from build123d import *

# Parameters (mm, degrees)
SKETCH_1_W               = 20
SKETCH_1_H               = 24
EXTRUDE_1_DEPTH          = 24
CUT_EXTRUDE_1_DEPTH      = 24
SKETCH_3_W               = 10
SKETCH_3_H               = 5
CUT_EXTRUDE_2_DEPTH      = 20
EXTRUDE_2_DEPTH          = 10
SKETCH_5_W               = 10
SKETCH_5_H               = 16
EXTRUDE_3_DEPTH          = 6
FILLET_2_R               = 0.5
CHAMFER_3_SIZE           = 3
CHAMFER_4_SIZE           = 3
FILLET_3_R               = 1
CUT_EXTRUDE_3_REACH      = 24
CUT_EXTRUDE_3_END_RADIUS = 5
CUT_EXTRUDE_4_REACH      = 20
CUT_EXTRUDE_4_END_RADIUS = 5
FILLET_6_R               = 3
FILLET_7_R               = 3


with BuildPart() as part:
    # 草图1 → 拉伸1 (new body)
    with BuildSketch(Plane.XY):
        with Locations((10, 12)):
            Rectangle(SKETCH_1_W, SKETCH_1_H)
    extrude(amount=EXTRUDE_1_DEPTH)

    # 草图2 → 切除-拉伸1 (cut)
    with BuildSketch(Plane.XY.offset(24)):
        with BuildLine():
            Line((6.75, 15.75), (6.75, 8.25))
            ThreePointArc((6.75, 8.25), (10, 5), (13.25, 8.25))
            Line((13.25, 8.25), (13.25, 15.75))
            ThreePointArc((13.25, 15.75), (10, 19), (6.75, 15.75))
        make_face()
    extrude(amount=-CUT_EXTRUDE_1_DEPTH, mode=Mode.SUBTRACT)

    # 草图3 → 切除-拉伸2 (cut)
    with BuildSketch(Plane(origin=(0, 24, 0), x_dir=(1, 0, 0), z_dir=(0, 1, 0))):
        with Locations((10, -12.5)):
            Rectangle(SKETCH_3_W, SKETCH_3_H)
    extrude(amount=-CUT_EXTRUDE_2_DEPTH, mode=Mode.SUBTRACT)

    # 草图4 → 拉伸2 (add)
    with BuildSketch(Plane.XZ):
        with BuildLine():
            Line((15, 19), (10, 19))
            ThreePointArc((10, 19), (6.464466094, 17.535533906), (5, 14))
            Line((5, 14), (5, 9))
            Line((5, 9), (10, 9))
            ThreePointArc((10, 9), (13.535533906, 10.464466094), (15, 14))
            Line((15, 14), (15, 19))
        make_face()
    extrude(amount=EXTRUDE_2_DEPTH)

    # 草图5 → 拉伸3 (add)
    with BuildSketch(Plane.XZ.offset(10)):
        with Locations((10, 14)):
            Rectangle(SKETCH_5_W, SKETCH_5_H)
    extrude(amount=-EXTRUDE_3_DEPTH)

    # 圆角2
    fillet_2_edges = [part.edges().sort_by_distance(p)[0] for p in [
        (20, 12, 24),
        (0, 12, 24),
        (20, 12, 0),
        (0, 12, 0),
    ]]
    fillet(fillet_2_edges, radius=FILLET_2_R)

    # 倒角3
    chamfer_3_edges = [part.edges().sort_by_distance(p)[0] for p in [
        (10, -10, 22),
    ]]
    chamfer(chamfer_3_edges, length=CHAMFER_3_SIZE)

    # 倒角4
    chamfer_4_edges = [part.edges().sort_by_distance(p)[0] for p in [
        (10, -10, 6),
    ]]
    chamfer(chamfer_4_edges, length=CHAMFER_4_SIZE)

    # 圆角3
    fillet_3_edges = [part.edges().sort_by_distance(p)[0] for p in [
        (10, -10, 19),
        (10, -10, 9),
    ]]
    fillet(fillet_3_edges, radius=FILLET_3_R)

    # 切除-拉伸3: up to this cylinder (the profile starts outside it)
    cut_extrude_3_end = Plane(origin=(10, -4.087346, 14), z_dir=(0, 1, 0)) * Cylinder(CUT_EXTRUDE_3_END_RADIUS, 59, mode=Mode.PRIVATE)
    # 草图8 → 切除-拉伸3 (cut, up to the surface)
    with BuildSketch(Plane.XY.offset(22), mode=Mode.PRIVATE) as cut_extrude_3_sk1:
        Polygon((10, -4), (5, -4), (5, -4.262038896), align=None)
    cut_extrude_3_tool1 = extrude(cut_extrude_3_sk1.sketch, amount=-CUT_EXTRUDE_3_REACH, mode=Mode.PRIVATE) - cut_extrude_3_end
    add(cut_extrude_3_tool1.solids().sort_by_distance((6.666667, -4.087346, 22))[0], mode=Mode.SUBTRACT)

    # 切除-拉伸4: up to this cylinder (the profile starts outside it)
    cut_extrude_4_end = Plane(origin=(10, -4.087346, 14), z_dir=(0, 1, 0)) * Cylinder(CUT_EXTRUDE_4_END_RADIUS, 51, mode=Mode.PRIVATE)
    # 草图9 → 切除-拉伸4 (cut, up to the surface)
    with BuildSketch(Plane(origin=(0, 0, 6), x_dir=(-1, 0, 0), z_dir=(0, 0, -1)), mode=Mode.PRIVATE) as cut_extrude_4_sk1:
        Polygon((-10, -4), (-15, -4), (-15, -4.262038896), align=None)
    cut_extrude_4_tool1 = extrude(cut_extrude_4_sk1.sketch, amount=-CUT_EXTRUDE_4_REACH, mode=Mode.PRIVATE) - cut_extrude_4_end
    add(cut_extrude_4_tool1.solids().sort_by_distance((13.333333, -4.087346, 6))[0], mode=Mode.SUBTRACT)

    # 圆角6
    fillet_6_edges = [part.edges().sort_by_distance(p)[0] for p in [
        (15, -5.631019448, 6),
    ]]
    fillet(fillet_6_edges, radius=FILLET_6_R)

    # 圆角7
    fillet_7_edges = [part.edges().sort_by_distance(p)[0] for p in [
        (5, -5.631019448, 22),
    ]]
    fillet(fillet_7_edges, radius=FILLET_7_R)


solid = part.part
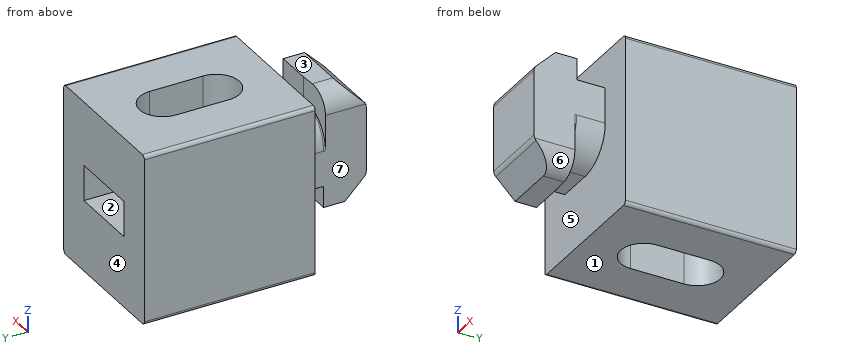
For this review, take the finished solid that the model builds, in its own axes (mm). Face numbers are marked on the shaded views. A direction names the side the tool comes from. Give positions to 0.01 mm unless a question says otherwise; leave off trailing zeros. Order: outer loops, then holes, each group sorted by start corner. A loop starts at its lowest first (then second) coordinate and runs counter-clockwise, first axis right, second up. Notation, with made-up numbers: (2.25, 47) -> (7.25, 47) arc R20 ccw to (7.25, 74) -> close; hole circle Ø1 at (30, 66). An arc over 180 degrees is marked (long way). Write item = value, one per line.
1) Draft analysis for pull direction Z (two halves, no side actions). For the marked faces 1, 2, 3 and 4, state which applies: pulls with the +Z half, pulls with the -Z half, needs draft (parallel to the pull), parting line crosses it, or undercut.
Findings:
face_1 = pulls with the -Z half
face_2 = undercut
face_3 = pulls with the +Z half
face_4 = needs draft
2) To check wall thickness, follow L1, parallel to X at y = 14.5, z = 6.5; L2, parallel to Z at x = 12.25, y = 18.5; L3, parallel to X at y = 16.5, z = 12.25. State the ranges of each line that lie inside material, in increasing order. Write a range as from..to.
Findings:
L1 = 0..6.75, 13.25..20
L2 = 0..10, 15..24
L3 = 0..5, 15..20
3) We need section D-D, the plane z = 2. Give the boundary of the cut face in (x, y), and give its area (3 significant figures).
Findings:
outline = (0, 0) -> (20, 0) -> (20, 24) -> (0, 24) -> close; hole (6.75, 8.25) arc R3.25 ccw to (13.25, 8.25) -> (13.25, 15.75) arc R3.25 ccw to (6.75, 15.75) -> close
area = 398 mm^2
4) We need section C-C, the plane x = 9.5. Give the boundary of the cut face in (y, z), and give its area (3 significant figures).
Findings:
outline = (-10, 9.41) arc R1 ccw to (-9.71, 8.71) -> (-7, 6) -> (-4, 6) -> (-4, 9) -> (0, 9) -> (0, 0) -> (5.04, 0) -> (5.04, 10) -> (4, 10) -> (4, 15) -> (5.04, 15) -> (5.04, 24) -> (0, 24) -> (0, 18.97) -> (-4.03, 18.97) -> (-4.03, 22) -> (-7, 22) -> (-9.71, 19.29) arc R1 ccw to (-10, 18.59) -> close; (18.96, 0) -> (24, 0) -> (24, 10) -> (18.96, 10) -> close; (18.96, 15) -> (24, 15) -> (24, 24) -> (18.96, 24) -> close
area = 338 mm^2
5) For the marked faces 5, 6 and 7, list the 3-axis set-ups (+Z, -Z, +X, -X, +Y, -Y) from which the entire face can be reached by the end or side of a thin tool; tool diameter is ignored.
Findings:
face_5 = none
face_6 = -Z, +X, -Y
face_7 = +Z, -Z, -X, -Y
6) We need section B-B, the plane z = 8. Give the boundary of the cut face in (x, y), and give its area (3 significant figures).
Findings:
outline = (0, 0) -> (20, 0) -> (20, 24) -> (0, 24) -> close; (5, -9) -> (14.83, -9) -> (14.83, -4.25) -> (10, -4) -> (5, -4) -> close; hole (6.75, 8.25) arc R3.25 ccw to (13.25, 8.25) -> (13.25, 15.75) arc R3.25 ccw to (6.75, 15.75) -> close
area = 447 mm^2
7) We need section A-A, the plane y = 15. Give the boundary of the cut face in (x, z).
Findings:
outline = (0, 0.5) arc R0.5 ccw to (0.5, 0) -> (6.75, 0) -> (6.75, 10) -> (5, 10) -> (5, 15) -> (6.75, 15) -> (6.75, 24) -> (0.5, 24) arc R0.5 ccw to (0, 23.5) -> close; (13.25, 0) -> (19.5, 0) arc R0.5 ccw to (20, 0.5) -> (20, 23.5) arc R0.5 ccw to (19.5, 24) -> (13.25, 24) -> (13.25, 15) -> (15, 15) -> (15, 10) -> (13.25, 10) -> close
8) Insertion check: pin 1 (3 mm diameter, centred on x = 11.5, y = -2, fed in from +Z); pin 2 (3 mm diameter, centred on x = 7.5, y = -2, fed in from -Z); pin 3 (2.5 mm diameter, centred on x = 10, y = -5.5, fed in from -Z). Each pin has a flat end and moves straight along its axis. Give the tip position at first contact, or say it passes through.
Findings:
pin_1 = 19
pin_2 = 9
pin_3 = 6
